```python
from build123d import *

# Parameters (mm, degrees)
F0_R         = 1.6
F0_R_2       = 1.25
F1_DEPTH     = 1
F2_T1_DEPTH  = 1
F2_T3_DEPTH  = 1
F2_T5_DEPTH  = 16
F2_T7_DEPTH  = 16
F2_T9_DEPTH  = 16
F2_T11_DEPTH = 16
F3_R         = 5


# Not quite as in the source:
# - a fillet or chamfer that OpenCascade refuses, or shapes differently, is made with other operations: its cross-section is extruded or revolved along the edge and cut away or added


with BuildPart() as f1:
    # F0 (on Top) → F1 (new body)
    with BuildSketch(Plane.XY):
        Polygon((15, -3.5), (15, 3.5), (5, 3.5), (-5, 3.5), (-15, 3.5), (-15, -3.5), (-5, -3.5), (-5, -2.5), (5, -2.5), (5, -3.5), align=None)
        with Locations((-9, -0.5)):
            Circle(F0_R, mode=Mode.SUBTRACT)
        with Locations((9, -0.5)):
            Circle(F0_R, mode=Mode.SUBTRACT)
        with Locations((0, 1)):
            Circle(F0_R_2, mode=Mode.SUBTRACT)
    extrude(amount=F1_DEPTH)

    # F2: fillet of radius 3 on 6 edges, made by hand

    # F2_s2 → F2_t1 (join)
    with BuildSketch(Plane.XY):
        with BuildLine():
            ThreePointArc((5, -3.5), (3.9886768939, -2.7613872125), (2.7639320225, -2.5))
            Line((2.7639320225, -2.5), (5, -2.5))
            Line((5, -2.5), (5, -3.5))
        make_face()
    extrude(amount=F2_T1_DEPTH)

    # F2_s4 → F2_t3 (join)
    with BuildSketch(Plane.XY):
        with BuildLine():
            ThreePointArc((-5, -3.5), (-3.9886768939, -2.7613872125), (-2.7639320225, -2.5))
            Line((-2.7639320225, -2.5), (-5, -2.5))
            Line((-5, -2.5), (-5, -3.5))
        make_face()
    extrude(amount=F2_T3_DEPTH)

    # F2_s6 → F2_t5 (cut)
    with BuildSketch(Plane.XY.offset(-7.5)):
        with BuildLine():
            ThreePointArc((15, -0.5), (14.1213203436, -2.6213203436), (12, -3.5))
            Line((12, -3.5), (15, -3.5))
            Line((15, -3.5), (15, -0.5))
        make_face()
    extrude(amount=F2_T5_DEPTH, mode=Mode.SUBTRACT)

    # F2_s8 → F2_t7 (cut)
    with BuildSketch(Plane.XY.offset(-7.5)):
        with BuildLine():
            ThreePointArc((15, 0.5), (14.1213203436, 2.6213203436), (12, 3.5))
            Line((12, 3.5), (15, 3.5))
            Line((15, 3.5), (15, 0.5))
        make_face()
    extrude(amount=F2_T7_DEPTH, mode=Mode.SUBTRACT)

    # F2_s10 → F2_t9 (cut)
    with BuildSketch(Plane.XY.offset(-7.5)):
        with BuildLine():
            ThreePointArc((-12, -3.5), (-14.1213203436, -2.6213203436), (-15, -0.5))
            Line((-15, -0.5), (-15, -3.5))
            Line((-15, -3.5), (-12, -3.5))
        make_face()
    extrude(amount=F2_T9_DEPTH, mode=Mode.SUBTRACT)

    # F2_s12 → F2_t11 (cut)
    with BuildSketch(Plane.XY.offset(-7.5)):
        with BuildLine():
            ThreePointArc((-15, 0.5), (-14.1213203436, 2.6213203436), (-12, 3.5))
            Line((-12, 3.5), (-15, 3.5))
            Line((-15, 3.5), (-15, 0.5))
        make_face()
    extrude(amount=F2_T11_DEPTH, mode=Mode.SUBTRACT)

    # F3
    f3_edges = [f1.edges().sort_by_distance(p)[0] for p in [
        (-5, -3.5, 0.5),
        (5, -3.5, 0.5),
    ]]
    fillet(f3_edges, radius=F3_R)


solid = f1.part
```
Check sheet for the modelled part. Datum: model origin and axes. Units: mm. A direction names the side the tool comes from. Give positions to 0.01 mm unless a question says otherwise; leave off trailing zeros. Order: outer loops, then holes, each group sorted by start corner. A loop starts at its lowest first (then second) coordinate and runs counter-clockwise, first axis right, second up. Notation, with made-up numbers: (-35, 27) -> (-8, 27) arc R24 cw to (-8, 48) -> close; hole circle Ø2 at (77.25, 25). An arc over 180 degrees is marked (long way). Use CSV: the item, a comma, the result in double quotes. Start each with the question number.
1) Material ranges on line 1 (Y direction, x = -9, z = 0.3); line 2 (Y direction, x = 0, z = 0.85); line 3 (X direction, y = 1.75, z = 0.1), recorded low to high. Write a range as from..to.
2) Sectioned sample at C-C, the plane y = -1.5. Record the boundary of the cut face in (x, z).
3) Set-up check for faces 1 (the face through (5.37, -3.337, 0.507)), 2 (the face through (-10.6, -0.43, 0.49)): record each of +Z, -Z, +X, -X, +Y, -Y from which the full face is reachable in a straight line by a thin tool's end or side.
4) Sectioned sample at A-A, the plane z = 0.6. Record the boundary of the cut face in (x, y) (3 decimals).
5) Go/stop test with a flat-tipped pin: P1, Ø4, axis at x = 9, y = -0.5, coming from the -Z side. Record where the tip stops, or that it passes through.
6) Sectioned sample at D-D, the plane y = 2. Record the boundary of the cut face in (x, z), plus the area to 3 significant figures.
7) Sectioned sample at B-B, the plane x = 9. Record the boundary of the cut face in (y, z), plus the area to 3 significant figures.
8) Mould release check, pull along Y, two halves, no side actions. Record for faces 3 (the face through (0, -1, 0)), 4 (the face through (-5.37, -3.337, 0.507)), 5 (the face through (-0.27, -0.22, 0.49)): released by +Y, released by -Y, zero draft, split by the parting line, or undercut.
Recorded:
1,line 1,"-3.5..-2.1, 1.1..3.5"
1,line 2,"-2.5..-0.25, 2.25..3.5"
1,line 3,"-14.73..-1, 1..14.73"
2,outline,"(-14.83, 0) -> (-10.25, 0) -> (-10.25, 1) -> (-14.83, 1) -> close; (-7.75, 0) -> (7.75, 0) -> (7.75, 1) -> (-7.75, 1) -> close; (10.25, 0) -> (14.83, 0) -> (14.83, 1) -> (10.25, 1) -> close"
3,face 1,"+Z, -Z, -Y"
3,face 2,"+Z, -Z"
4,outline,"(-15, -0.5) arc R3 ccw to (-12, -3.5) -> (-6.637, -3.5) arc R5 ccw to (-4.216, -2.875) arc R3 cw to (-2.764, -2.5) -> (2.764, -2.5) arc R3 cw to (4.216, -2.875) arc R5 ccw to (6.637, -3.5) -> (12, -3.5) arc R3 ccw to (15, -0.5) -> (15, 0.5) arc R3 ccw to (12, 3.5) -> (-12, 3.5) arc R3 ccw to (-15, 0.5) -> close; hole circle Ø3.2 at (-9, -0.5); hole circle Ø2.5 at (0, 1); hole circle Ø3.2 at (9, -0.5)"
5,P1,"z = 0"
6,outline,"(-14.6, 0) -> (-0.75, 0) -> (-0.75, 1) -> (-14.6, 1) -> close; (0.75, 0) -> (14.6, 0) -> (14.6, 1) -> (0.75, 1) -> close"
6,area,"27.7 mm2"
7,outline,"(-3.5, 0) -> (-2.1, 0) -> (-2.1, 1) -> (-3.5, 1) -> close; (1.1, 0) -> (3.5, 0) -> (3.5, 1) -> (1.1, 1) -> close"
7,area,"3.80 mm2"
8,face 3,"zero draft"
8,face 4,"released by -Y"
8,face 5,"undercut"
